```python
from build123d import *

# Parameters (mm, degrees)
SKETCH1_W           = 10
SKETCH1_H           = 55
BOSS_EXTRUDE1_DEPTH = 30
BOSS_EXTRUDE2_START = -27.5
BOSS_EXTRUDE2_DEPTH = 10
FILLET3_R           = 5
FILLET4_R           = 5
SKETCH3_R           = 15
BOSS_EXTRUDE3_DEPTH = 25
HOLE1_D             = 20
FILLET5_R           = 5
HOLE2_D             = 5
BOSS_EXTRUDE7_DEPTH = 2


with BuildPart() as part:
    # Sketch1 → Boss-Extrude1 (new, symmetric)
    with BuildSketch(Plane.XY):
        Rectangle(SKETCH1_W, SKETCH1_H)
    extrude(amount=BOSS_EXTRUDE1_DEPTH, both=True)

    # Sketch2 → Boss-Extrude2 (add)
    with BuildSketch(Plane(origin=(0, 0, 0), x_dir=(1, 0, 0), z_dir=(0, 1, 0)).offset(BOSS_EXTRUDE2_START)):
        with BuildLine():
            Line((65, 25), (3, 25))
            Line((3, 25), (3, -25))
            Line((3, -25), (65, -25))
            ThreePointArc((65, -25), (90, 0), (65, 25))
        make_face()
    extrude(amount=BOSS_EXTRUDE2_DEPTH)

    # Fillet3
    fillet3_edges = [part.edges().sort_by_distance(p)[0] for p in [
        (5, -22.5, 25),
    ]]
    fillet(fillet3_edges, radius=FILLET3_R - 0.0001)  # a hair under: the kernel refuses the full size

    # Fillet4
    fillet4_edges = [part.edges().sort_by_distance(p)[0] for p in [
        (5, -22.5, -25),
    ]]
    fillet(fillet4_edges, radius=FILLET4_R - 0.0001)  # a hair under: the kernel refuses the full size

    # Sketch3 → Boss-Extrude3 (add)
    with BuildSketch(Plane(origin=(0, -17.5, 0), x_dir=(1, 0, 0), z_dir=(0, 1, 0))):
        with Locations(Location((65, 0, 0), (0, 0, 270))):
            Circle(SKETCH3_R)
    extrude(amount=BOSS_EXTRUDE3_DEPTH)

    # Hole1 (through all)
    with Locations(Plane(origin=(0, 7.5, 0), x_dir=(1, 0, 0), z_dir=(0, 1, 0))):
        with Locations((65, 0)):
            Hole(HOLE1_D / 2)

    # Fillet5
    fillet5_edges = [part.edges().sort_by_distance(p)[0] for p in [
        (0, 27.5, -30),
        (0, 27.5, 30),
    ]]
    fillet(fillet5_edges, radius=FILLET5_R)

    # Hole2 (through all)
    with Locations(Plane(origin=(5, 0, 0), x_dir=(0, 0, -1), z_dir=(1, 0, 0))):
        with Locations((-25, 22.5), (25, 22.5)):
            Hole(HOLE2_D / 2)

    # Sketch9 → Boss-Extrude7 (add, symmetric)
    with BuildSketch(Plane.XY):
        with BuildLine():
            Line((51.5, 7.5), (51.5, -17.5))
            Line((51.5, -17.5), (10, -17.5))
            Line((10, -17.5), (5, -17.5))
            Line((5, -17.5), (3, -17.5))
            Line((3, -17.5), (3, 27.5))
            Line((3, 27.5), (5, 27.5))
            ThreePointArc((5, 27.5), (25.683225718, 13.412257866), (50, 7.5))
            Line((50, 7.5), (51.5, 7.5))
        make_face()
    extrude(amount=BOSS_EXTRUDE7_DEPTH, both=True)


solid = part.part
```
Source: CAD feature listing. Evaluate the final solid. Frame: model axes, mm. A direction names the side the tool comes from. Round coordinates to 2 decimals unless told otherwise and drop trailing zeros. Loops run counter-clockwise (first coordinate to the right, second up) from the corner with the lowest first, then second, coordinate; pieces in that order, holes last.
1. Contact query for flat-ended pins moving along their axis: pin 1 (18 mm diameter, centred on x = 65, z = 0, fed in from -Y); pin 2 (3 mm diameter, centred on x = 40, y = -21.5, fed in from -Z); pin 3 (22.5 mm diameter, centred on x = 25, y = 10, fed in from +Z); pin 4 (8 mm diameter, centred on x = 36.5, z = 24, fed in from +Y). Output: stop coordinate, or through.
2. Ray query, L1, parallel to Y at x = 2.75, z = -25; L2, parallel to Z at x = 0, y = 22; L3, parallel to Z at x = 16, y = -10. Return the intervals inside material, ascending.
3. Section query C-C on x = 15.5. Output: boundary loops of the cut face in (y, z).
4. Section query A-A on z = 0. Output: boundary loops of the cut face in (x, y), and give its area (3 significant figures).
5. Access query for faces 4 (the flat face through (47, -17.5, -7)), 5 (the flat face through (62, 7.5, 10)), 6 (the flat face through (37, -23, 25)). Directions: +Z, -Z, +X, -X, +Y, -Y. A direction counts if a zero-diameter tool reaches every point of the face in a straight line with its end or side. Return the directions, or none.
6. Section query B-B on y = -9.5. Output: boundary loops of the cut face in (x, z), and give its area (3 significant figures).
7. Mould query, pull axis X, two halves, no side actions, for faces 1 (the cylindrical face through (0, 25, 25)), 2 (the cylindrical face through (89.994, -22.57, 0.55)), 3 (the flat face through (5, 6, 16)). Classes: released by +X, released by -X, zero draft, split by the parting line, or undercut.
Answers below:
1. pin 1: passes through
1. pin 2: stops at z = -25
1. pin 3: stops at z = 2
1. pin 4: stops at y = -17.5
2. L1: y = -27.5 to 20, 25 to 27.5
2. L2: z = -30 to -27.45, -22.55 to 22.55, 27.45 to 30
2. L3: z = -2 to 2
3. outline: (-27.5, -25) - (-17.5, -25) - (-17.5, -2) - (18.99, -2) - (18.99, 2) - (-17.5, 2) - (-17.5, 25) - (-27.5, 25) - close
4. outline: (-5, -27.5) - (55, -27.5) - (55, 7.5) - (50, 7.5) arc R70 cw to (5, 27.5) - (-5, 27.5) - close; (75, -27.5) - (90, -27.5) - (90, -17.5) - (80, -17.5) - (80, 7.5) - (75, 7.5) - close
4. area: 2,880 mm2
5. face 4: +Y
5. face 5: +Z, -Z, +X, +Y
5. face 6: +Z, +X, +Y, -Y
6. outline: (-5, -30) - (5, -30) - (5, -2) - (50.13, -2) arc R15 ccw (long way) to (50.13, 2) - (5, 2) - (5, 30) - (-5, 30) - close; hole circle Ø20 at (65, 0)
6. area: 1,170 mm2
7. face 1: zero draft
7. face 2: released by +X
7. face 3: undercut
